```python
from build123d import *

# Parameters (mm, degrees)
SKETCH_1_W          = 40
SKETCH_1_H          = 40
EXTRUDE_1_DEPTH     = 5
CHAMFER_1_SIZE      = 3
SKETCH_2_R          = 10
EXTRUDE_2_DEPTH     = 2
SKETCH_3_R          = 6
EXTRUDE_3_DEPTH     = 22
SKETCH_4_R          = 6
SKETCH_4_R_2        = 5.5
CUT_EXTRUDE_1_DEPTH = 3
SKETCH_5_R          = 2.5
CUT_EXTRUDE_2_DEPTH = 38.094473982
CHAMFER_2_SIZE      = 3
CHAMFER_3_SIZE      = 0.5


with BuildPart() as part:
    # Эскиз1 → Бобышка-Вытянуть1 (new body)
    with BuildSketch(Plane(origin=(0, 0, 0), x_dir=(1, 0, 0), z_dir=(0, 1, 0))):
        Rectangle(SKETCH_1_W, SKETCH_1_H)
    extrude(amount=EXTRUDE_1_DEPTH)

    # Фаска1
    chamfer_1_edges = [part.edges().sort_by_distance(p)[0] for p in [
        (20, 2.5, 20),
        (-20, 2.5, 20),
        (-20, 2.5, -20),
        (20, 2.5, -20),
    ]]
    chamfer(chamfer_1_edges, length=CHAMFER_1_SIZE)

    # Эскиз2 → Бобышка-Вытянуть2 (add)
    with BuildSketch(Plane(origin=(0, 5, 0), x_dir=(1, 0, 0), z_dir=(0, 1, 0))):
        with Locations(Location((0, 0, 0), (0, 0, 270))):
            Circle(SKETCH_2_R)
    extrude(amount=EXTRUDE_2_DEPTH)

    # Эскиз3 → Бобышка-Вытянуть3 (add)
    with BuildSketch(Plane(origin=(0, 7, 0), x_dir=(1, 0, 0), z_dir=(0, 1, 0))):
        with Locations(Location((0, 0, 0), (0, 0, 270))):
            Circle(SKETCH_3_R)
    extrude(amount=EXTRUDE_3_DEPTH)

    # Эскиз4 → Вырез-Вытянуть1 (cut)
    with BuildSketch(Plane(origin=(0, 7, 0), x_dir=(1, 0, 0), z_dir=(0, 1, 0))):
        with Locations(Location((0, 0, 0), (0, 0, 270))):
            Circle(SKETCH_4_R)
        with Locations(Location((0, 0, 0), (0, 0, 270))):
            Circle(SKETCH_4_R_2, mode=Mode.SUBTRACT)
    extrude(amount=CUT_EXTRUDE_1_DEPTH, mode=Mode.SUBTRACT)

    # Эскиз5 → Вырез-Вытянуть2 (cut, through all)
    with BuildSketch(Plane(origin=(0, 5, 0), x_dir=(1, 0, 0), z_dir=(0, 1, 0))):
        with Locations(Location((-12.5, 12.5, 0), (0, 0, 270))):
            Circle(SKETCH_5_R)
        with Locations(Location((12.5, 12.5, 0), (0, 0, 270))):
            Circle(SKETCH_5_R)
        with Locations(Location((12.5, -12.5, 0), (0, 0, 270))):
            Circle(SKETCH_5_R)
        with Locations(Location((-12.5, -12.5, 0), (0, 0, 270))):
            Circle(SKETCH_5_R)
    extrude(amount=-CUT_EXTRUDE_2_DEPTH, mode=Mode.SUBTRACT)

    # Фаска2
    chamfer_2_edges = [part.edges().sort_by_distance(p)[0] for p in [
        (-12.5, 5, 10),
        (12.5, 5, 10),
        (12.5, 5, -15),
        (-12.5, 5, -15),
    ]]
    chamfer(chamfer_2_edges, length=CHAMFER_2_SIZE)

    # Фаска3
    chamfer_3_edges = [part.edges().sort_by_distance(p)[0] for p in [
        (0, 29, -6),
    ]]
    chamfer(chamfer_3_edges, length=CHAMFER_3_SIZE)


solid = part.part
```
Model file for the job. Use its own axes, mm. A direction names the side the tool comes from. Round coordinates to 2 decimals unless told otherwise and drop trailing zeros. Write each loop counter-clockwise with the first axis right and the second up, starting at its lowest first coordinate (ties: lowest second). Pieces come first, ordered by that corner, then holes. Notation, with made-up numbers: M 12,-12.5 L 51,-12.5 A19 cw 51,-2.5 Z; hole C 75.25,40.5 d10. An arc over 180 degrees is marked long. Put each result on its own line as item: value.
Item 1: Probe L1, parallel to X at y = 0.65, z = -12.5; L2, parallel to Y at x = -14, z = 1; L3, parallel to Y at x = 1, z = 6.5. List the from-to ranges inside material, lowest first. Write a range as from..to.
Responses:
L1: -20..-15, -10..10, 15..20
L2: 0..5
L3: 0..7
Item 2: Cut at A-A (x = -12.5). List the corners of the cut face in (y, z).
Responses:
outline: M 0,-20 L 5,-20 L 5,-18 L 2,-15 L 0,-15 Z; M 0,-10 L 2,-10 L 5,-7 L 5,7 L 2,10 L 0,10 Z; M 0,15 L 2,15 L 5,18 L 5,20 L 0,20 Z
Item 3: Cut at B-B (z = -12.5). List the corners of the cut face in (x, y), and give its area (3 significant figures).
Responses:
outline: M -20,0 L -15,0 L -15,2 L -18,5 L -20,5 Z; M -10,0 L 10,0 L 10,2 L 7,5 L -7,5 L -10,2 Z; M 15,0 L 20,0 L 20,5 L 18,5 L 15,2 Z
area: 132 mm²
Item 4: Mould opens along Y. For faces 1 (the flat face through (20, 2, 0)), 2 (the flat face through (-5, 10, 3)), 3 (the conical face through (-10.269, 2.146, -11.078)) say: +Y half, -Y half, draft (parallel to the pull), parting line (faces both ways), or undercut.
Responses:
face 1: draft
face 2: undercut
face 3: +Y half
Item 5: Flat gauge pins, fed straight in: P1, Ø6, axis at x = 7.5, z = -8.5, coming from the +Y side; P2, Ø1.5, axis at x = 10.5, z = 4.5, coming from the +Y side; P3, Ø8, axis at y = 10, z = 6, coming from the -X side. Where does each tip first touch, or does it go through?
Responses:
P1: y = 7
P2: y = 5
P3: x = -9.42
Item 6: Cut at D-D (x = 0). List the corners of the cut face in (y, z), and give its area (3 significant figures).
Responses:
outline: M 0,-20 L 5,-20 L 5,-10 L 7,-10 L 7,-5.5 L 10,-5.5 L 10,-6 L 28.5,-6 L 29,-5.5 L 29,5.5 L 28.5,6 L 10,6 L 10,5.5 L 7,5.5 L 7,10 L 5,10 L 5,20 L 0,20 Z
area: 501 mm²
Item 7: Tool access for faces 4 (the flat face through (0, 29, 0)), 5 (the flat face through (-5, 5, -9)): list every direction of +Z, -Z, +X, -X, +Y, -Y with a clear straight run to the whole face (end or side of a thin tool).
Responses:
face 4: +Z, -Z, +X, -X, +Y
face 5: +Y
Item 8: Cut at C-C (z = 0). List the corners of the cut face in (x, y), and give its area (3 significant figures).
Responses:
outline: M -20,0 L 20,0 L 20,5 L 10,5 L 10,7 L 5.5,7 L 5.5,10 L 6,10 L 6,28.5 L 5.5,29 L -5.5,29 L -6,28.5 L -6,10 L -5.5,10 L -5.5,7 L -10,7 L -10,5 L -20,5 Z
area: 501 mm²
